```python
from build123d import *

# Parameters (mm, degrees)
BOSS_EXTRUDE1_DEPTH = 3.175


with BuildPart() as part:
    # Sketch3 → Boss-Extrude1 (new body)
    with BuildSketch(Plane(origin=(0, 0, 0), x_dir=(1, 0, 0), z_dir=(0, 1, 0))):
        with BuildLine():
            Line((-5.541525375, 3.58326618), (-2.47962532, 5.150959008))
            Line((-2.47962532, 5.150959008), (-2.47962532, 6.474170352))
            ThreePointArc((-2.47962532, 6.474170352), (-2.221563685, 14.417025562), (4.617359972, 10.369227654))
            ThreePointArc((4.617359972, 10.369227654), (4.047797908, 8.147663968), (2.47962532, 6.474170352))
            Line((2.47962532, 6.474170352), (2.47962532, 5.20231788))
            Line((2.47962532, 5.20231788), (5.873962228, 3.007468661))
            Line((5.873962228, 3.007468661), (5.541525375, -3.58326618))
            Line((5.541525375, -3.58326618), (4.701204968, -4.013510228))
            Line((4.701204968, -4.013510228), (4.701204968, -6.905610932))
            Line((4.701204968, -6.905610932), (5.918780254, -8.378526195))
            ThreePointArc((5.918780254, -8.378526195), (9.922634137, -0.265088751), (6.526624698, 8.120961152))
            ThreePointArc((6.526624698, 8.120961152), (5.706991897, 14.686716316), (0, 18.035026682))
            ThreePointArc((0, 18.035026682), (-5.706991897, 14.686716316), (-6.526624698, 8.120961152))
            ThreePointArc((-6.526624698, 8.120961152), (-9.922634137, -0.265088751), (-5.918780254, -8.378526195))
            Line((-5.918780254, -8.378526195), (-4.701204968, -6.905610932))
            Line((-4.701204968, -6.905610932), (-4.701204968, -3.765798027))
            Line((-4.701204968, -3.765798027), (-5.873962228, -3.007468661))
            Line((-5.873962228, -3.007468661), (-5.541525375, 3.58326618))
        make_face()
        with BuildLine():
            Line((-2.47962532, 6.474170352), (-2.47962532, 5.150959008))
            Line((-2.47962532, 5.150959008), (-1.063503338, 5.876013463))
            ThreePointArc((-1.063503338, 5.876013463), (-1.79663243, 6.115743784), (-2.47962532, 6.474170352))
        make_face()
        with BuildLine():
            ThreePointArc((2.47962532, 6.474170352), (1.921985685, 6.17089654), (1.328021538, 5.946968965))
            Line((1.328021538, 5.946968965), (2.47962532, 5.20231788))
            Line((2.47962532, 5.20231788), (2.47962532, 6.474170352))
        make_face()
    extrude(amount=BOSS_EXTRUDE1_DEPTH)

    # Fillet6
    # a fillet whose section is not a circle: 1.27 mm, written as the material it takes off along each edge
    with BuildSketch(Plane(origin=(1.328021538, -5.283304691, -5.946968965), x_dir=(0.8397378391322112, 0, 0.5429920455490709), z_dir=(0, 1, 0))) as fillet6_piece_1:
        with BuildLine():
            Bezier((2.113321876, 0), (0.3966534, 0), (0.898889741, 1.641556979), weights=[1, 0.118948346, 1])
            ThreePointArc((0.898889741, 1.641556979), (0.533488386, 0.774757636), (0, 0))
            Line((0, 0), (2.113321876, 0))
        make_face()
    extrude(amount=13.741609382, mode=Mode.SUBTRACT)
    with BuildSketch(Plane(origin=(-1.063503338, -6.120582224, -5.876013463), x_dir=(-0.891835980226881, 0, -0.4523589110128793), z_dir=(0, 1, 0))) as fillet6_piece_2:
        with BuildLine():
            Bezier((2.168149873, 0), (0.323600022, 0.445521101), (1.438773255, 1.980852292), weights=[1, 0.11123936, 1])
            Line((1.438773255, 1.980852292), (0, 0))
            ThreePointArc((0, 0), (1.084074937, 0.129064678), (2.168149873, 0))
        make_face()
    extrude(amount=15.416164449, mode=Mode.SUBTRACT)


solid = part.part
```
Geometry: final body of the model. Coordinates: model frame, mm. A direction names the side the tool comes from. Give positions to 0.01 mm unless a question says otherwise; leave off trailing zeros. Write each loop counter-clockwise with the first axis right and the second up, starting at its lowest first coordinate (ties: lowest second). Pieces come first, ordered by that corner, then holes.
1. Line query: probe 1 along X at (y, z) = (0.55, -12.25); probe 2 along X at (y, z) = (0.3, 6); probe 3 along Z at (x, y) = (3.75, 2.15). Output: solid intervals per line, ascending.
2. Section query A-A, the plane z = -7.25. Return loops of the section in (x, y) (3 decimals), then the cut area to 3 significant figures.
3. Section query B-B, the plane z = -4. Return loops of the section in (x, y) (3 decimals).
4. Pin query (flat end, axial travel): P1, Ø1.5, axis at y = 1.5, z = -9, coming from the +X side; P2, Ø1, axis at x = 5, y = 2, coming from the +Z side; P3, Ø6, axis at x = 7, z = -10, coming from the -Y side; P4, Ø0.9, axis at y = 2, z = 5, coming from the +X side. Return the tip coordinate at first contact, or that it passes through.
5. Section query C-C, the plane x = -1. Return loops of the section in (y, z) (3 decimals).
6. Reachability of faces 5 (the flat face through (-5.28, 1.57, 3.39)), 6 (the flat face through (4, 0, -6)), 7 (the flat face through (5.3, 1.57, 7.63)) from +Z, -Z, +X, -X, +Y, -Y: full face, straight path, thin tool, end or side. Return the list, or none.
7. Draft query along X for faces 1 (the cylindrical face through (5.759, 1.565, -14.606)), 2 (the cylindrical face through (-5.65, 1.57, -14.77)), 3 (the flat face through (5.71, 1.57, 0.24)), 4 (the flat face through (-4.701, 2, 5)). Return one class per face: released by +X, released by -X, zero draft, split by the parting line, or undercut.
Computed:
1. probe 1: x = -6.75 to -4.22, 4.22 to 6.75
1. probe 2: x = -8.07 to -4.7, 4.7 to 8.07
1. probe 3: z = -16.7 to -13.06, -7.68 to -4.38
2. outline: (-7.342, 0) - (-3.404, 0) - (-3.404, 3.175) - (-7.342, 3.175) - close; (3.404, 0) - (7.342, 0) - (7.342, 3.175) - (3.404, 3.175) - close
2. area: 25.0 mm2
3. outline: (-9.235, 0) - (-4.728, 0) - (-4.728, 3.175) - (-9.235, 3.175) - close; (4.339, 0) - (9.235, 0) - (9.235, 3.175) - (4.339, 3.175) - close
4. P1: stops at x = 6.89
4. P2: stops at z = 7.87
4. P3: stops at y = 0
4. P4: stops at x = 8.89
5. outline: (0, -17.894) - (3.175, -17.894) - (3.175, -14.877) - (0, -14.877) - close
6. face 5: +Y, -Y
6. face 6: +Z, -Z, +X, -X, -Y
6. face 7: +Z, +Y, -Y
7. face 1: released by +X
7. face 2: released by -X
7. face 3: undercut
7. face 4: undercut
